Build history of the part. All positions in model axes, mm. A direction names the side the tool comes from. Coordinates: 2 decimals unless noted, no trailing zeros. Loops run counter-clockwise (first coordinate to the right, second up) from the corner with the lowest first, then second, coordinate; pieces in that order, holes last.
Item 1: Cut at B-B (z = -5.75). List the corners of the cut face in (x, y), and give its area (3 significant figures).
Item 2: Cut at A-A (y = 228.75). List the corners of the cut face in (x, z), and give its area (3 significant figures).
Item 3: Mould opens along Y. For faces 1 (the face through (8.897, 14.638, -19.24)), 2 (the face through (1, 0, -10)), 3 (the face through (20, 128, -10)) say: released by +Y, released by -Y, zero draft, split by the parting line, or undercut.
Item 4: Cut at D-D (y = 71.5). List the corners of the cut face in (x, z), and give its area (3 significant figures).
Item 5: Cut at C-C (x = 11). Count the separate pieces of the cut face and the enclosed holes in it, and give its area (3 significant figures).
Item 6: Drill centre lines: line 1 along Y through (x, z) = (11, -0.8); line 2 along X through (y, z) = (143.5, -10); line 3 along Z through (x, y) = (11.25, 111.5). Where is each one in solid material? Low to high.
Item 7: Flat gauge pins, fed straight in: pin 1 (3 mm diameter, centred on x = 12.5, z = -16.5, fed in from +Y); pin 2 (6 mm diameter, centred on x = 11, y = 228.75, fed in from +Z). Where does each tip first touch, or does it go through?
Item 8: 3-axis set-ups, long thin cutter, end or side, ignore diameter. For faces 4 (the face through (7.13, 247.3, -0.74)), 5 (the face through (18.5, 128, -10)), 6 (the face through (10.66, 231.38, -19.24)): which of +Z, -Z, +X, -X, +Y, -Y reach the whole face in a straight line?
from build123d import *

# Parameters (mm, degrees)
SKETCH1_W           = 17
SKETCH1_H           = 17
BOSS_EXTRUDE1_DEPTH = 260
SKETCH2_R           = 2.65
CUT_EXTRUDE1_DEPTH  = 262.533936612
SKETCH3_R           = 5.25
CUT_EXTRUDE2_DEPTH  = 10


with BuildPart() as part:
    # Sketch1 → Boss-Extrude1 (new body)
    with BuildSketch(Plane(origin=(0, 0, 0), x_dir=(1, 0, 0), z_dir=(0, 1, 0))):
        with BuildLine():
            Line((0.5, 0), (19.5, 0))
            ThreePointArc((19.5, 0), (19.853553391, 0.146446609), (20, 0.5))
            Line((20, 0.5), (20, 19.5))
            ThreePointArc((20, 19.5), (19.853553391, 19.853553391), (19.5, 20))
            Line((19.5, 20), (0.5, 20))
            ThreePointArc((0.5, 20), (0.146446609, 19.853553391), (0, 19.5))
            Line((0, 19.5), (0, 0.5))
            ThreePointArc((0, 0.5), (0.146446609, 0.146446609), (0.5, 0))
        make_face()
        with Locations((10, 10)):
            Rectangle(SKETCH1_W, SKETCH1_H, mode=Mode.SUBTRACT)
    extrude(amount=BOSS_EXTRUDE1_DEPTH)

    # Sketch2 → Cut-Extrude1 (cut, through all)
    with BuildSketch(Plane.XY):
        with Locations((11, 243.75)):
            Circle(SKETCH2_R)
        with Locations((11, 228.75)):
            Circle(SKETCH2_R)
        with Locations((11, 31.25)):
            Circle(SKETCH2_R)
        with Locations((11, 16.25)):
            Circle(SKETCH2_R)
    extrude(amount=-CUT_EXTRUDE1_DEPTH, mode=Mode.SUBTRACT)

    # Sketch3 → Cut-Extrude2 (cut)
    with BuildSketch(Plane.XY):
        with Locations((11, 243.75)):
            Circle(SKETCH3_R)
        with Locations((11, 228.75)):
            Circle(SKETCH3_R)
        with Locations((11, 31.25)):
            Circle(SKETCH3_R)
        with Locations((11, 16.25)):
            Circle(SKETCH3_R)
    extrude(amount=-CUT_EXTRUDE2_DEPTH, mode=Mode.SUBTRACT)


solid = part.part
Filled sheet:
1. outline: (0, 0) - (1.5, 0) - (1.5, 260) - (0, 260) - close; (18.5, 0) - (20, 0) - (20, 260) - (18.5, 260) - close
1. area: 780 mm2
2. outline: (0, -19.5) arc R0.5 ccw to (0.5, -20) - (8.35, -20) - (8.35, -18.5) - (1.5, -18.5) - (1.5, -1.5) - (5.75, -1.5) - (5.75, 0) - (0.5, 0) arc R0.5 ccw to (0, -0.5) - close; (13.65, -20) - (19.5, -20) arc R0.5 ccw to (20, -19.5) - (20, -0.5) arc R0.5 ccw to (19.5, 0) - (16.25, 0) - (16.25, -1.5) - (18.5, -1.5) - (18.5, -18.5) - (13.65, -18.5) - close
2. area: 87.1 mm2
3. face 1: undercut
3. face 2: released by -Y
3. face 3: zero draft
4. outline: (0, -19.5) arc R0.5 ccw to (0.5, -20) - (19.5, -20) arc R0.5 ccw to (20, -19.5) - (20, -0.5) arc R0.5 ccw to (19.5, 0) - (0.5, 0) arc R0.5 ccw to (0, -0.5) - close; hole (1.5, -18.5) - (18.5, -18.5) - (18.5, -1.5) - (1.5, -1.5) - close
4. area: 111 mm2
5. separate pieces: 10
5. enclosed holes: 0
5. area: 685 mm2
6. line 1: y = 0 to 11, 21.5 to 26, 36.5 to 223.5, 234 to 238.5, 249 to 260
6. line 2: x = 0 to 1.5, 18.5 to 20
6. line 3: z = -20 to -18.5, -1.5 to 0
7. pin 1: passes through
7. pin 2: stops at z = -18.5
8. face 4: +Z
8. face 5: +Y, -Y
8. face 6: +Z, -Z
